Can you work these out from the drawing? Everything is in mm from the part's minimum corner. Coordinates: 2 decimals unless noted, no trailing zeros. Order: outer loops, then holes, each group sorted by start corner. A loop starts at its lowest first (then second) coordinate and runs counter-clockwise, first axis right, second up. Notation, with made-up numbers: (52, 88) -> (61, 88) arc R26 ccw to (61, 120) -> close; hole circle Ø7 at (-1.75, 31). An arc over 180 degrees is marked (long way). Put each result on its own line as item: value. Start each with the question number.
Q1. If we section it at C-C (y = 75): Please give me the cut outline in (x, z).
Q2. If we section it at A-A (x = 3.3): Please give me the cut outline in (y, z).
Q3. If we section it at D-D (y = 122): Please give me the cut outline in (x, z), and give its area (3 significant figures).
Q4. Please list where these lines run through material, in increasing order: line 1 along Z through (x, y) = (2.95, 75); line 2 along Z through (x, y) = (1.1, 75); line 3 along Z through (x, y) = (3.75, 31).
Q5. Will this pin go through, and if not, where does the flat tip stop? pin 1 (4 mm diameter, centred on y = 47.5, z = 65.5, fed in from +X).
Q6. If we section it at B-B (z = 60): Please give me the cut outline in (x, y).
Q7. We'd pull the mould along Z, two halves only. Please class the marked faces 1 and 2: +Z half, -Z half, draft (parallel to the pull), parting line (faces both ways), or undercut.
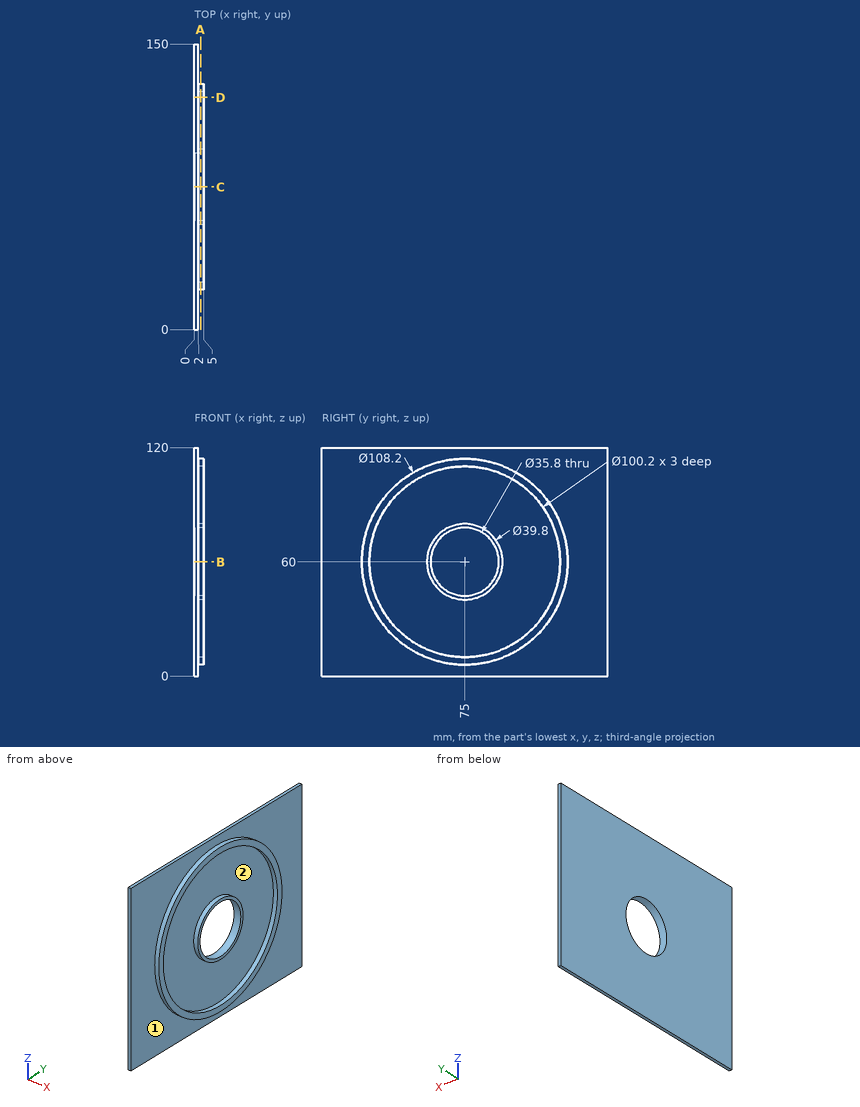
The answers:
1. outline: (0, 0) -> (2, 0) -> (2, 5.9) -> (5, 5.9) -> (5, 9.9) -> (2, 9.9) -> (2, 40.1) -> (5, 40.1) -> (5, 42.1) -> (0, 42.1) -> close; (0, 77.9) -> (5, 77.9) -> (5, 79.9) -> (2, 79.9) -> (2, 110.1) -> (5, 110.1) -> (5, 114.1) -> (2, 114.1) -> (2, 120) -> (0, 120) -> close
2. outline: circle Ø108.2 at (75, 60); circle Ø39.8 at (75, 60); hole circle Ø100.2 at (75, 60); hole circle Ø35.8 at (75, 60)
3. outline: (0, 0) -> (2, 0) -> (2, 33.21) -> (5, 33.21) -> (5, 42.65) -> (2, 42.65) -> (2, 77.35) -> (5, 77.35) -> (5, 86.79) -> (2, 86.79) -> (2, 120) -> (0, 120) -> close
3. area: 297 mm^2
4. line 1: 5.9 to 9.9, 40.1 to 42.1, 77.9 to 79.9, 110.1 to 114.1
4. line 2: 0 to 42.1, 77.9 to 120
4. line 3: 28.52 to 36.04, 83.96 to 91.48
5. pin 1: x = 2
6. outline: (0, 0) -> (2, 0) -> (2, 20.9) -> (5, 20.9) -> (5, 24.9) -> (2, 24.9) -> (2, 55.1) -> (5, 55.1) -> (5, 57.1) -> (0, 57.1) -> close; (0, 92.9) -> (5, 92.9) -> (5, 94.9) -> (2, 94.9) -> (2, 125.1) -> (5, 125.1) -> (5, 129.1) -> (2, 129.1) -> (2, 150) -> (0, 150) -> close
7. face 1: draft
7. face 2: undercut
